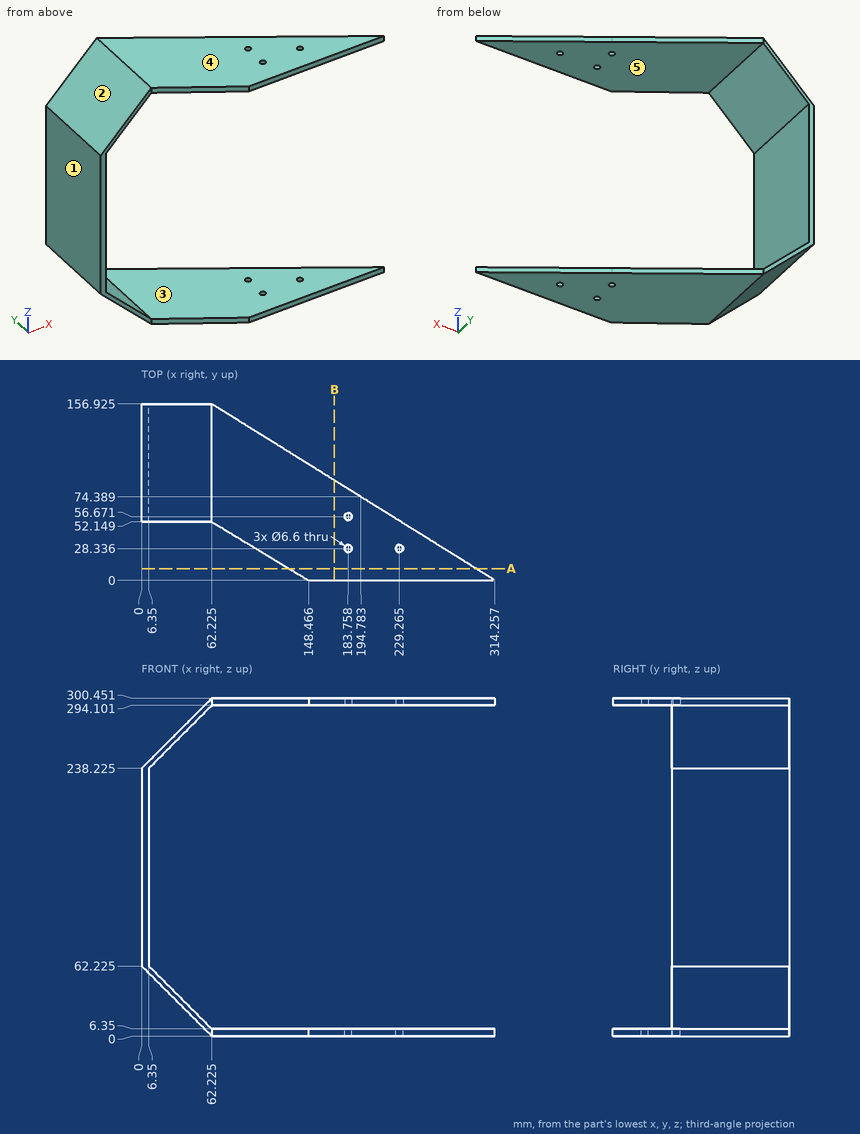
Geometry check sheet. Reference: drawing and pictorial views, mm from the part's lowest x, y, z. A direction names the side the tool comes from. Round coordinates to 2 decimals unless told otherwise and drop trailing zeros. Write each loop counter-clockwise with the first axis right and the second up, starting at its lowest first coordinate (ties: lowest second). Pieces come first, ordered by that corner, then holes.
(1) Access from +Z, -Z, +X, -X, +Y, -Y to the whole of each face (thin tool, end or side, straight path). Record for the marked faces 4 and 5.
Returned:
face 4: +Z, +X, -X, +Y, -Y
face 5: +X, +Y, -Y
(2) Section check B-B (x = 171.5). Enter the section's corners in (y, z).
Returned:
outline: (0, 0) - (88.89, 0) - (88.89, 6.35) - (0, 6.35) - close; (0, 294.1) - (88.89, 294.1) - (88.89, 300.45) - (0, 300.45) - close
(3) Depth check by flat-ended pin: pin 1 Ø1 at (x, y) = (48, 83) entering from -Z (1 decimal); pin 2 Ø2 at (y, z) = (126, 57) entering from +X (1 decimal); pin 3 Ø4 at (x, y) = (183.76, 28.34) entering from +Z. Enter the tip coordinate at first touch or a pass-through.
Returned:
pin 1: stops at z = 13.7
pin 2: stops at x = 12.6
pin 3: passes through
(4) Section check A-A (y = 10.5). Enter the section's corners in (x, z), plus the area to 3 significant figures.
Returned:
outline: (131.1, 0) - (297.39, 0) - (297.39, 6.35) - (131.1, 6.35) - close; (131.1, 294.1) - (297.39, 294.1) - (297.39, 300.45) - (131.1, 300.45) - close
area: 2,110 mm2
(5) Material ranges on line 1 (Z direction, x = 125, y = 43.5); line 2 (X direction, y = 128, z = 142.5); line 3 (Z direction, x = 49.5, y = 56) (1 decimal), recorded low to high.
Returned:
line 1: z = 0 to 6.35, 294.1 to 300.45
line 2: x = 0 to 6.35
line 3: z = 12.7 to 19.1, 281.4 to 287.7
(6) Mould release check, pull along Z, two halves, no side actions. Record for the marked faces 1, 2 and 3: pulls with the +Z half, pulls with the -Z half, needs draft (parallel to the pull), parting line crosses it, or undercut.
Returned:
face 1: needs draft
face 2: pulls with the +Z half
face 3: undercut
